Here's how the part is built. I have some questions about the finished solid (model axes, mm). A direction names the side the tool comes from. Round coordinates to 2 decimals unless told otherwise and drop trailing zeros. Order: outer loops, then holes, each group sorted by start corner. A loop starts at its lowest first (then second) coordinate and runs counter-clockwise, first axis right, second up. Notation, with made-up numbers: M 68.25,22 L 72.25,22 A27 cw 72.25,60 Z; hole C 28,-17.75 d7. An arc over 180 degrees is marked long. Write item = value, one per line. Start each with the question number.
Item 1: I'm going to push flat-ended pins straight in: P1, Ø0.5, axis at x = 9, z = 32.5, coming from the -Y side; P2, Ø1.5, axis at y = 1, z = 41, coming from the -X side; P3, Ø0.9, axis at y = 9, z = 48.5, coming from the +X side. Where does each tip first touch, or does it pass through?
Item 2: Please list where these lines run through material, in increasing order: L1, parallel to Y at x = 0, z = 26.5; L2, parallel to X at y = 5.5, z = 67; L3, parallel to X at y = 5.75, z = 15.
Item 3: I want a section at A-A, the plane x = 0. List the corners of the cut face in (y, z) for me.
Item 4: For faces 4 (the face through (0, 3.7, 43)), 5 (the face through (-9, 2.5, 43)), 6 (the face through (0, -3.7, 43)), 7 (the face through (4.226, -5.919, 43.095)), which set-ups out of +Z, -Z, +X, -X, +Y, -Y let a thin tool reach every point of the face, with its end or its side?
Item 5: We'd pull the mould along X, two halves only. Please class faces 1 (the face through (9.4, -9.43, 41.9)), 2 (the face through (9, 2.5, 43)), 3 (the face through (4, 8.2, 43)): pulls with the +X half, pulls with the -X half, needs draft (parallel to the pull), parting line crosses it, or undercut.
```python
from build123d import *

# Parameters (mm, degrees)
EXTRUSION1_DEPTH        = 85
PER_AGE1_OUTLINE_R      = 2.1
PER_AGE1_DEPTH          = 85
ENL_V_MAT_EXTRU_1_DEPTH = 300
ENL_V_MAT_EXTRU_3_DEPTH = 300
ENL_V_MAT_EXTRU_4_DEPTH = 87.168439698
ENL_V_MAT_EXTRU_7_DEPTH = 87.168439698


# Read off the part's stored shape, not the designer's step: Perçage1
with BuildPart() as part:
    # Esquisse1 → Extrusion1 (new body)
    with BuildSketch(Plane.XY):
        with BuildLine():
            Line((-10, 8), (-10, -8))
            ThreePointArc((-10, -8), (-9.414213562, -9.414213562), (-8, -10))
            Line((-8, -10), (8, -10))
            ThreePointArc((8, -10), (9.414213562, -9.414213562), (10, -8))
            Line((10, -8), (10, 8))
            ThreePointArc((10, 8), (9.414213562, 9.414213562), (8, 10))
            Line((8, 10), (-8, 10))
            ThreePointArc((-8, 10), (-9.414213562, 9.414213562), (-10, 8))
        make_face()
    extrude(amount=EXTRUSION1_DEPTH)

    # Perçage1 outline → Perçage1 (cut)
    with BuildSketch(Plane.XY):
        Circle(PER_AGE1_OUTLINE_R)
    extrude(amount=PER_AGE1_DEPTH, mode=Mode.SUBTRACT)

    # Esquisse3 → Enlèv. mat.-Extru.1 (cut)
    with BuildSketch(Plane.XY.offset(85)):
        Polygon((10, 2.5), (8.2, 2.5), (8.2, 6), (3.7, 2.5), (3.7, -2.5), (8.2, -6), (8.2, -2.5), (10, -2.5), align=None)
    extrude(amount=-ENL_V_MAT_EXTRU_1_DEPTH, mode=Mode.SUBTRACT)

    # Esquisse5 → Enlèv. mat.-Extru.3 (cut)
    with BuildSketch(Plane.XY.offset(85)):
        Polygon((-2.5, 10), (-2.5, 8.2), (-6, 8.2), (-2.5, 3.7), (2.5, 3.7), (6, 8.2), (2.5, 8.2), (2.5, 10), align=None)
    extrude(amount=-ENL_V_MAT_EXTRU_3_DEPTH, mode=Mode.SUBTRACT)

    # Esquisse6 → Enlèv. mat.-Extru.4 (cut, through all)
    with BuildSketch(Plane.XY.offset(85)):
        Polygon((-2.5, -10), (-2.5, -8.2), (-6, -8.2), (-2.5, -3.7), (2.5, -3.7), (6, -8.2), (2.5, -8.2), (2.5, -10), align=None)
    extrude(amount=-ENL_V_MAT_EXTRU_4_DEPTH, mode=Mode.SUBTRACT)

    # Esquisse4 → Enlèv. mat.-Extru.7 (cut, through all)
    with BuildSketch(Plane.XY.offset(85)):
        Polygon((-10, 2.5), (-8.2, 2.5), (-8.2, 6), (-3.7, 2.5), (-3.7, -2.5), (-8.2, -6), (-8.2, -2.5), (-10, -2.5), align=None)
    extrude(amount=-ENL_V_MAT_EXTRU_7_DEPTH, mode=Mode.SUBTRACT)


solid = part.part
```
Filled in:
q1.P1 = -9.85
q1.P2 = -3.7
q1.P3 = 9.92
q2.L1 = -3.7 to -2.1, 2.1 to 3.7
q2.L2 = -10 to -8.2, -7.56 to -3.9, 3.9 to 7.56, 8.2 to 10
q2.L3 = -10 to -8.2, -7.88 to -4.09, 4.09 to 7.88, 8.2 to 10
q3.outline = M -3.7,0 L -2.1,0 L -2.1,85 L -3.7,85 Z; M 2.1,0 L 3.7,0 L 3.7,85 L 2.1,85 Z
q4.face_4 = +Z, -Z, +Y
q4.face_5 = +Z, -Z, -X
q4.face_6 = +Z, -Z, -Y
q4.face_7 = +Z, -Z
q5.face_1 = pulls with the +X half
q5.face_2 = needs draft
q5.face_3 = undercut
